from build123d import *

# Parameters (mm, degrees)
F0_W     = 203.2
F0_H     = 76.2
F1_DEPTH = 76.2
F2_SIZE  = 10.16
F3_SIZE  = 5.07999
F4_R     = 12.7
F5_DEPTH = 50.8


# Not quite as in the source:
# - a fillet or chamfer is up to 0.001 mm smaller than in the source, because OpenCascade refuses the exact size


with BuildPart() as f1:
    # F0 (on Front) → F1 (new body)
    with BuildSketch(Plane.XZ):
        with Locations((4.1285920888, -9.8249100385)):
            Rectangle(F0_W, F0_H)
    extrude(amount=F1_DEPTH)

    # F2
    f2_edges = [f1.edges().sort_by_distance(p)[0] for p in [
        (4.128592, -76.2, 28.27509),
        (4.128592, -76.2, -47.92491),
        (4.128592, 0, 28.27509),
        (4.128592, 0, -47.92491),
    ]]
    chamfer(f2_edges, length=F2_SIZE)

    # F3 (size 5.08 in the source; OpenCascade refuses exactly that, so slightly less here)
    f3_edges = [f1.edges().sort_by_distance(p)[0] for p in [
        (-97.471408, -38.1, 28.27509),
        (-97.471408, -76.2, -9.82491),
        (-97.471408, -38.1, -47.92491),
        (-97.471408, 0, -9.82491),
        (105.728592, 0, -9.82491),
        (105.728592, -38.1, -47.92491),
        (105.728592, -76.2, -9.82491),
        (105.728592, -38.1, 28.27509),
    ]]
    chamfer(f3_edges, length=F3_SIZE)

    # F4 (on face) → F5 (cut)
    with BuildSketch(Plane(origin=(0, 0, -47.9249100385), x_dir=(1, 0, 0), z_dir=(0, 0, -1))):
        with Locations((0, 38.1)):
            Circle(F4_R)
    extrude(amount=-F5_DEPTH, mode=Mode.SUBTRACT)


solid = f1.part
CAD build for the part. Positions are in the model's coordinates, mm. A direction names the side the tool comes from. Round coordinates to 2 decimals unless told otherwise and drop trailing zeros. Loops run counter-clockwise (first coordinate to the right, second up) from the corner with the lowest first, then second, coordinate; pieces in that order, holes last. Notation, with made-up numbers: (35, 30.5) - (71, 30.5) arc R19 cw to (71, 36.5) - close; hole circle Ø8 at (55, 28). An arc over 180 degrees is marked (long way). Put each result on its own line as item: value.
1. 3-axis set-ups, long thin cutter, end or side, ignore diameter. For faces 1 (the flat face through (103.224, -2.576, -10.287)), 2 (the cylindrical face through (6.827, -48.809, -22.881)): which of +Z, -Z, +X, -X, +Y, -Y reach the whole face in a straight line?
Geometry check:
face 1: +Z, -Z, +X, +Y
face 2: -Z
2. Two-plate mould, pull along X, no slides. Class faces 3 (the flat face through (2.706, -71.191, -42.774)), 4 (the flat face through (-97.471, -38, -10)), 5 (the flat face through (0, -38, 2.875)): released by +X, released by -X, zero draft, split by the parting line, or undercut.
Geometry check:
face 3: zero draft
face 4: released by -X
face 5: undercut
3. Slice it at D-D on x = -24. List the corners of the cut face in (y, z).
Geometry check:
outline: (-76.2, -37.76) - (-66.04, -47.92) - (-10.16, -47.92) - (0, -37.76) - (0, 18.12) - (-10.16, 28.28) - (-66.04, 28.28) - (-76.2, 18.12) - close
4. Slice it at B-B on y = -38.1. List the corners of the cut face in (x, z).
Geometry check:
outline: (-97.47, -42.84) - (-92.39, -47.92) - (-12.7, -47.92) - (-12.7, 2.88) - (12.7, 2.88) - (12.7, -47.92) - (100.65, -47.92) - (105.73, -42.84) - (105.73, 23.2) - (100.65, 28.28) - (-92.39, 28.28) - (-97.47, 23.2) - close
5. Slice it at C-C on x = 0. List the corners of the cut face in (y, z).
Geometry check:
outline: (-76.2, -37.76) - (-66.04, -47.92) - (-50.8, -47.92) - (-50.8, 2.88) - (-25.4, 2.88) - (-25.4, -47.92) - (-10.16, -47.92) - (0, -37.76) - (0, 18.12) - (-10.16, 28.28) - (-66.04, 28.28) - (-76.2, 18.12) - close
6. Slice it at A-A on z = -5.5. List the corners of the cut face in (x, y).
Geometry check:
outline: (-97.47, -71.12) - (-92.39, -76.2) - (100.65, -76.2) - (105.73, -71.12) - (105.73, -5.08) - (100.65, 0) - (-92.39, 0) - (-97.47, -5.08) - close; hole circle Ø25.4 at (0, -38.1)
7. Wall check: line 1 (Y direction, x = 0, z = -19); line 2 (X direction, y = -38, z = -21); line 3 (X direction, y = -31, z = -23). Give the ranges that are in metal, low to high.
Geometry check:
line 1: -76.2 to -50.8, -25.4 to 0
line 2: -97.47 to -12.7, 12.7 to 105.73
line 3: -97.47 to -10.53, 10.53 to 105.73
8. Pin check, flat tip, straight feed: P1, Ø15, axis at x = 0, y = -38.1, coming from the -Z side. Stop position of the tip, or through.
Geometry check:
P1: z = 2.88
